Design review of the part built by this model. Coordinates are the model's own, in mm. A direction names the side the tool comes from. Round coordinates to 2 decimals unless told otherwise and drop trailing zeros. Order: outer loops, then holes, each group sorted by start corner. A loop starts at its lowest first (then second) coordinate and runs counter-clockwise, first axis right, second up.
from build123d import *

# Parameters (mm, degrees)
PAD_DEPTH   = 3
FILLET_R    = 1
FILLET001_R = 2.5


with BuildPart() as part:
    # Sketch → Pad (new body)
    with BuildSketch(Plane.XY):
        Polygon((13.058418, 32.987703), (13.058418, -7.012297), (9.808418, -7.012297), (9.808418, -10.012297), (-0.091582, -10.012297), (-0.091582, -7.012297), (-40.191582, -7.012297), (-40.191582, -10.012297), (-50.091582, -10.012297), (-50.091582, -7.012297), (-53.341582, -7.012297), (-53.341582, 32.987703), (-50.091582, 32.987703), (-50.091582, 35.987703), (-40.191582, 35.987703), (-40.191582, 32.987703), (-0.091582, 32.987703), (-0.091582, 35.987703), (9.808418, 35.987703), (9.808418, 32.987703), align=None)
    extrude(amount=PAD_DEPTH)

    # Fillet
    fillet_edges = [part.edges().sort_by_distance(p)[0] for p in [
        (-50.091582, 35.987703, 1.5),
        (-40.191582, 35.987703, 1.5),
        (-0.091582, 35.987703, 1.5),
        (9.808418, 35.987703, 1.5),
        (9.808418, -10.012297, 1.5),
        (-0.091582, -10.012297, 1.5),
        (-40.191582, -10.012297, 1.5),
        (-50.091582, -10.012297, 1.5),
    ]]
    fillet(fillet_edges, radius=FILLET_R)

    # Fillet001
    fillet001_edges = [part.edges().sort_by_distance(p)[0] for p in [
        (-53.341582, 32.987703, 1.5),
        (-53.341582, -7.012297, 1.5),
        (13.058418, 32.987703, 1.5),
        (13.058418, -7.012297, 1.5),
    ]]
    fillet(fillet001_edges, radius=FILLET001_R)


with BuildPart() as part_1:
    # Fillet001 placement: moved
    add(part.part.moved(Location((200, 100, 0))))


solid = part_1.part
1) Take a section at B-B on x = 182. Give the boundary of the cut face in (y, z), plus the area to 3 significant figures.
Results:
outline: (92.99, 0) - (132.99, 0) - (132.99, 3) - (92.99, 3) - close
area: 120 mm2
2) For faces 1 (the face through (149.908, 134, 1)), 2 (the face through (199.908, 92, 1)), 3 (the face through (209.808, 92, 1)), 4 (the face through (159.808, 134, 1)), list the 3-axis set-ups (+Z, -Z, +X, -X, +Y, -Y) from which the entire face can be reached by the end or side of a thin tool; tool diameter is ignored.
Results:
face 1: +Z, -Z, -X, +Y
face 2: +Z, -Z, -Y
face 3: +Z, -Z, +X, -Y
face 4: +Z, -Z, +Y
3) To check wall thickness, follow line 1 along Y through (x, z) = (179, 0.7). State the ranges of the line that lie inside material, in increasing order.
Results:
line 1: y = 92.99 to 132.99
4) Clearance check with flat-ended pins moving along their axes: P1, Ø1, axis at y = 92, z = 1, coming from the -X side; P2, Ø1.5, axis at x = 195, z = 2, coming from the +Y side; P3, Ø1.6, axis at y = 134, z = 2, coming from the +X side; P4, Ø10, axis at x = 170.5, y = 124, coming from the -Z side. State where each tip first meets the part, or that it passes through.
Results:
P1: stops at x = 149.91
P2: stops at y = 132.99
P3: stops at x = 209.81
P4: stops at z = 0
